Geometry check sheet. Reference: the model listing, model coordinates, mm. A direction names the side the tool comes from. Give positions to 0.01 mm unless a question says otherwise; leave off trailing zeros. Order: outer loops, then holes, each group sorted by start corner. A loop starts at its lowest first (then second) coordinate and runs counter-clockwise, first axis right, second up.
from build123d import *

# Parameters (mm, degrees)
SKETCH_1_W          = 9.5
SKETCH_1_H          = 45
EXTRUDE_1_DEPTH     = 5.5
SKETCH_2_W          = 3
SKETCH_2_H          = 37
CUT_EXTRUDE_1_DEPTH = 3
SKETCH_3_R          = 1.1
CUT_EXTRUDE_2_DEPTH = 3
SKETCH_4_W          = 1
SKETCH_4_H          = 0.5
EXTRUDE_2_DEPTH     = 4


with BuildPart() as part:
    # 草图1 → 凸台-拉伸1 (new body)
    with BuildSketch(Plane(origin=(0, 0, 0), x_dir=(1, 0, 0), z_dir=(0, 1, 0))):
        Rectangle(SKETCH_1_W, SKETCH_1_H)
    extrude(amount=EXTRUDE_1_DEPTH)

    # 草图2 → 切除-拉伸1 (cut)
    with BuildSketch(Plane(origin=(0, 5.5, 0), x_dir=(1, 0, 0), z_dir=(0, 1, 0))):
        Rectangle(SKETCH_2_W, SKETCH_2_H)
    extrude(amount=-CUT_EXTRUDE_1_DEPTH, mode=Mode.SUBTRACT)

    # 草图3 → 切除-拉伸2 (cut)
    with BuildSketch(Plane(origin=(0, 5.5, 0), x_dir=(1, 0, 0), z_dir=(0, 1, 0))):
        with Locations(Location((0, -20.5, 0), (0, 0, 270))):
            Circle(SKETCH_3_R)
        with Locations(Location((0, 20.5, 0), (0, 0, 90))):
            Circle(SKETCH_3_R)
    extrude(amount=-CUT_EXTRUDE_2_DEPTH, mode=Mode.SUBTRACT)

    # 草图4 → 凸台-拉伸2 (add)
    with BuildSketch(Plane.XZ):
        with Locations((2, 22.25)):
            Rectangle(SKETCH_4_W, SKETCH_4_H)
        with Locations((-2, 22.25)):
            Rectangle(SKETCH_4_W, SKETCH_4_H)
        with Locations((2, -22.25)):
            Rectangle(SKETCH_4_W, SKETCH_4_H)
    extrude(amount=EXTRUDE_2_DEPTH)


solid = part.part
Item 1: Sectioned sample at C-C (y = -3). Enter the section's corners in (x, z), and give its area (3 significant figures).
Reported:
outline: (-2.5, 22) - (-1.5, 22) - (-1.5, 22.5) - (-2.5, 22.5) - close; (1.5, -22.5) - (2.5, -22.5) - (2.5, -22) - (1.5, -22) - close; (1.5, 22) - (2.5, 22) - (2.5, 22.5) - (1.5, 22.5) - close
area: 1.50 mm2
Item 2: Set-up check for faces 1 (the flat face through (2, -2, -22)), 2 (the flat face through (-2, -2, 22)), 3 (the flat face through (4.75, 3, 0)), 4 (the flat face through (0, 3, -22.5)), 5 (the flat face through (-1.5, 4, 0)): record each of +Z, -Z, +X, -X, +Y, -Y from which the full face is reachable in a straight line by a thin tool's end or side.
Reported:
face 1: +X, -X, -Y
face 2: -Z, +X, -X, -Y
face 3: +Z, -Z, +X, +Y, -Y
face 4: -Z, +X, -X, +Y, -Y
face 5: +Y
Item 3: Scan lines: L1, parallel to X at y = 5, z = -3; L2, parallel to X at y = 3.9, z = -20.5; L3, parallel to Y at x = -1.25, z = 15. Record each from-to range of solid material in increasing order.
Reported:
L1: x = -4.75 to -1.5, 1.5 to 4.75
L2: x = -4.75 to -1.1, 1.1 to 4.75
L3: y = 0 to 2.5
Item 4: Sectioned sample at A-A (y = 3). Enter the section's corners in (x, z), and give its area (3 significant figures).
Reported:
outline: (-4.75, -22.5) - (4.75, -22.5) - (4.75, 22.5) - (-4.75, 22.5) - close; hole (-1.5, -18.5) - (1.5, -18.5) - (1.5, 18.5) - (-1.5, 18.5) - close; hole circle Ø2.2 at (0, -20.5); hole circle Ø2.2 at (0, 20.5)
area: 309 mm2
Item 5: Sectioned sample at B-B (z = -12.5). Enter the section's corners in (x, y), and give its area (4 significant figures).
Reported:
outline: (-4.75, 0) - (4.75, 0) - (4.75, 5.5) - (1.5, 5.5) - (1.5, 2.5) - (-1.5, 2.5) - (-1.5, 5.5) - (-4.75, 5.5) - close
area: 43.25 mm2
Item 6: Gauge pin test, flat ends, axial feed: pin 1 (2 mm diameter, centred on x = 0, z = -10.5, fed in from +Y); pin 2 (0.6 mm diameter, centred on y = -3, z = -22, fed in from -X). Record the tip position at first contact, or that the pin passes through.
Reported:
pin 1: stops at y = 2.5
pin 2: stops at x = 1.5
Item 7: Sectioned sample at D-D (x = 0). Enter the section's corners in (y, z), and give its area (3 significant figures).
Reported:
outline: (0, -22.5) - (5.5, -22.5) - (5.5, -21.6) - (2.5, -21.6) - (2.5, -19.4) - (5.5, -19.4) - (5.5, -18.5) - (2.5, -18.5) - (2.5, 18.5) - (5.5, 18.5) - (5.5, 19.4) - (2.5, 19.4) - (2.5, 21.6) - (5.5, 21.6) - (5.5, 22.5) - (0, 22.5) - close
area: 123 mm2
